from build123d import *

# Parameters (mm, degrees)
SKETCH1_W                                         = 250
SKETCH1_H                                         = 150
BOSS_EXTRUDE1_DEPTH                               = 5
CUT_EXTRUDE1_DEPTH                                = 5
CSK_FOR_8_FLAT_HEAD_MACHINE_SCREW_100_D           = 4.4958
CSK_FOR_8_FLAT_HEAD_MACHINE_SCREW_100_CSINK_D     = 8.4328
CSK_FOR_8_FLAT_HEAD_MACHINE_SCREW_100_CSINK_ANGLE = 100
CHAMFER1_SIZE                                     = 2


with BuildPart() as part:
    # Sketch1 → Boss-Extrude1 (new body)
    with BuildSketch(Plane(origin=(0, 0, 0), x_dir=(1, 0, 0), z_dir=(0, 1, 0))):
        with Locations((125, 75)):
            Rectangle(SKETCH1_W, SKETCH1_H)
    extrude(amount=BOSS_EXTRUDE1_DEPTH)

    # Sketch2 → Cut-Extrude1 (cut)
    with BuildSketch(Plane(origin=(0, 5, 0), x_dir=(1, 0, 0), z_dir=(0, 1, 0))):
        Polygon((5, 5), (245, 5), (245, 68.522708921), (235, 68.522708921), (235, 81.477291079), (245, 81.477291079), (245, 145), (5, 145), align=None)
    extrude(amount=-CUT_EXTRUDE1_DEPTH, mode=Mode.SUBTRACT)

    # CSK for #8 Flat Head Machine Screw (100)1 (through all)
    with Locations(Plane(origin=(240.110859841, 5, -75.135992341), x_dir=(0, 0, 1), z_dir=(0, 1, 0))):
        with Locations((0, 0)):
            CounterSinkHole(CSK_FOR_8_FLAT_HEAD_MACHINE_SCREW_100_D / 2, CSK_FOR_8_FLAT_HEAD_MACHINE_SCREW_100_CSINK_D / 2, counter_sink_angle=CSK_FOR_8_FLAT_HEAD_MACHINE_SCREW_100_CSINK_ANGLE)

    # Chamfer1
    chamfer1_edges = [part.edges().sort_by_distance(p)[0] for p in [
        (240.110859841, 0, -72.888092341),
    ]]
    chamfer(chamfer1_edges, length=CHAMFER1_SIZE)


solid = part.part
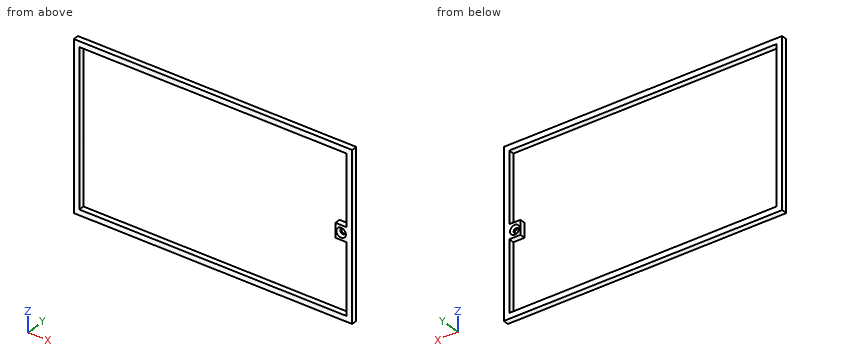
Read the model definition and answer for the solid it produces. Units are mm, in the model's axes. Round coordinates to 2 decimals unless told otherwise and drop trailing zeros. Order: outer loops, then holes, each group sorted by start corner. A loop starts at its lowest first (then second) coordinate and runs counter-clockwise, first axis right, second up. Notation, with made-up numbers: (-10, 49) - (20, 49) arc R20 cw to (20, 67) - close; hole circle Ø6 at (-6.5, -27). An arc over 180 degrees is marked (long way). Use one line per item in the form item = value. Start each with the question number.
(1) The part is cut by section A-A (z = -32.5). Give the vertices of the cut face in (x, y), then the cut area to 3 significant figures.
(2) A flat-ended cylindrical pin translates along its axis: pin 1 Ø5 at (x, z) = (240.11, -75.14) entering from +Y. Find the tip coordinate at first contact, or state that the pin passes through.
(3) The part is cut by section B-B (x = 221). Give the vertices of the cut face in (y, z), then the cut area to 3 significant figures.
(4) The part is cut by section C-C (y = 4.2). Give the vertices of the cut face in (x, z).
(5) Find the intervals of material crossed by line 1 along X through (y, z) = (2.5, -68); line 2 along X through (y, z) = (3.95, -70); line 3 along Z through (x, y) = (212, 4.4), in increasing order. Write a range as from..to.
Checked values:
q1.outline = (0, 0) - (5, 0) - (5, 5) - (0, 5) - close; (245, 0) - (250, 0) - (250, 5) - (245, 5) - close
q1.area = 50.0 mm^2
q2.pin_1 = 3.56
q3.outline = (0, -150) - (5, -150) - (5, -145) - (0, -145) - close; (0, -5) - (5, -5) - (5, 0) - (0, 0) - close
q3.area = 50.0 mm^2
q4.outline = (0, -150) - (250, -150) - (250, 0) - (0, 0) - close; hole (5, -145) - (245, -145) - (245, -81.48) - (235, -81.48) - (235, -68.52) - (245, -68.52) - (245, -5) - (5, -5) - close; hole circle Ø6.53 at (240.11, -75.14)
q5.line_1 = 0..5, 245..250
q5.line_2 = 0..5, 235..250
q5.line_3 = -150..-145, -5..0
